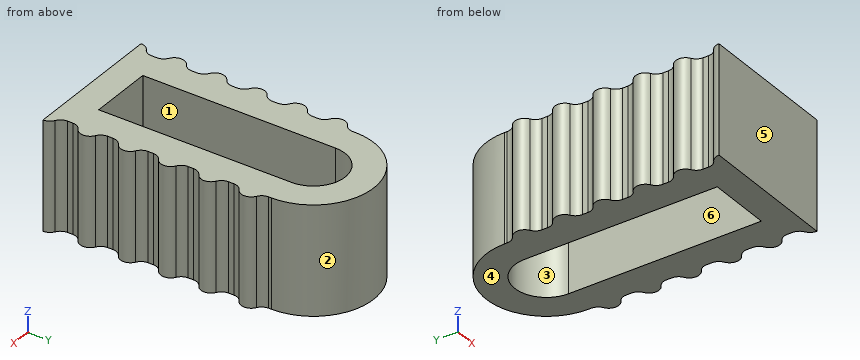
Autodesk Inventor part; units mm, degrees
ref_plane "Plan de construction1" through (3.5, 4, -2.7) normal (0, -1, 0) x (1, 0, 0)
ref_plane "YZ Plane" through (0, 0, 0) normal (1, 0, 0) x (0, 1, 0)
ref_plane "XZ Plane" through (0, 0, 0) normal (0, 1, 0) x (-1, 0, 0)
sketch "Esquisse1" plane through (0, 0, 0) normal (0, 0, 1) x (1, 0, 0)
  line L0 (-3, -7) -> (3, -7)
  line L1 (3, -7) -> (3, 4)
  line L2 (0, 7) -> (0, 7)
  line L3 (-3, 4) -> (-3, -7)
  line L4 (-3, -7) -> (3, 7) construction
  line L5 (3, -7) -> (-3, 7) construction
  arc A0 (0, 7) -> (-3, 4) centre (0, 4) ccw
  arc A1 (3, 4) -> (0, 7) centre (0, 4) ccw
  point P0 (0, 0)
  dimension "d0" = 6
  dimension "d1" = 14
  dimension "d2" = 3
extrude "Extrusion1" add sketch "Esquisse1" along normal mid plane 5.4
sketch "Esquisse2" plane through (0, 0, 2.7) normal (0, 0, 1) x (1, 0, 0)
  line L0 (-3, -7) -> (3, -7) construction
  line L1 (3, -7) -> (3, 4) construction
  arc A0 (3, 4) -> (-3, 4) centre (0, 4) ccw construction
  line L2 (-3, 4) -> (-3, -7) construction
  arc A1 (1.575, 4) -> (-1.575, 4) centre (0, 4) ccw
  line L3 (1.575, 4) -> (1.575, -5.575)
  line L4 (1.575, -5.575) -> (-1.575, -5.575)
  line L5 (-1.575, -5.575) -> (-1.575, 4)
  point P0 (0, 0)
  dimension "d21" = 3.15
extrude "Extrusion2" cut sketch "Esquisse2" against normal through all
sketch "Esquisse3" plane through (0, 0, 2.7) normal (0, 0, 1) x (1, 0, 0)
  line L0 (3, 4) -> (3, -7)
  arc A0 (3.5, -7) -> (3, -6.5) centre (3, -7) ccw
  line L1 (-3, -7) -> (3, -7)
  line L2 (3, -7) -> (3.5, -7)
  line L3 (3, -7) -> (3, -6.5)
  arc A1 (3, -5.5) -> (3, -4.5) centre (3, -5) ccw
  arc A2 (3, -3.5) -> (3, -2.5) centre (3, -3) ccw
  arc A3 (3, -1.5) -> (3, -0.5) centre (3, -1) ccw
  arc A4 (3, 0.5) -> (3, 1.5) centre (3, 1) ccw
  arc A5 (3, 2.5) -> (3, 3.5) centre (3, 3) ccw
  line L4 (3, -5.5) -> (3, -4.5)
  line L5 (3, -3.5) -> (3, -2.5)
  line L6 (3, -1.5) -> (3, -0.5)
  line L7 (3, 0.5) -> (3, 1.5)
  line L8 (3, 2.5) -> (3, 3.5)
  point P0 (0, 0)
  dimension "d8" = 1
  dimension "d9" = 1
  dimension "d10" = 2
  dimension "d13" = 2
extrude "Extrusion3" add sketch "Esquisse3" against normal up to surface (5.4 mm away)
mirror "Symétrie1" about plane through (0, 0, 0) normal (1, 0, 0) of "Extrusion3"
fillet "Congé1" radius 0.5 33 edges at (3, -6.5, -1.35) (3, -6.5, 1.35) (3, -5.5, -1.35) (3, -4.5, -1.35) (3, -5.5, 1.35) (3, -4.5, 1.35) (3, -3.5, -1.35) (3, -2.5, -1.35) (3, -3.5, 1.35) (3, -2.5, 1.35) (3, -1.5, -1.35) (3, -0.5, -1.35) (3, -1.5, 1.35) (3, -0.5, 1.35) (3, 0.5, -1.35) (3, 1.5, -1.35) (3, 0.5, 1.35) (3, 1.5, 1.35) (3, 2.5, -1.35) (3, 3.5, -1.35) (3, 2.5, 1.35) (3, 3.5, 1.35) (-3, -6.5, 0) (-3, -4.5, 0) (-3, -5.5, 0) (-3, -2.5, 0) (-3, -3.5, 0) (-3, -0.5, 0) (-3, -1.5, 0) (-3, 1.5, 0) (-3, 0.5, 0) (-3, 3.5, 0) (-3, 2.5, 0)
ref_plane "Plan de construction1" through (3.5, 4, -2.7) normal (0, -1, 0) x (1, 0, 0)
equation "\"d9\" = d8"
properties part number "Tendeur" material "Aluminium"
Geometry check sheet. Reference: the model listing, model coordinates, mm. Face numbers are marked on the shaded views. A direction names the side the tool comes from. Give positions to 0.01 mm unless a question says otherwise; leave off trailing zeros. Order: outer loops, then holes, each group sorted by start corner. A loop starts at its lowest first (then second) coordinate and runs counter-clockwise, first axis right, second up. Notation, with made-up numbers: (-23.75, -40) - (16.25, -40) arc R15 ccw to (16.25, -13) - close; hole circle Ø7 at (-29.75, 8.5). An arc over 180 degrees is marked (long way). Write item = value, one per line. Start each with the question number.
1) Scan lines: L1, parallel to Y at x = 0, z = 2.35 (3 decimals); L2, parallel to Y at x = 3.25, z = 0.8; L3, parallel to X at y = -5, z = -1.4 (3 decimals). Record each from-to range of solid material in increasing order.
2) Section check D-D (x = 2). Enter the section's corners in (y, z), then the cut area to 3 significant figures.
3) Section check C-C (x = -2.5). Enter the section's corners in (y, z), then the cut area to 3 significant figures.
4) Section check B-B (x = 0). Enter the section's corners in (y, z) (3 decimals), then the cut area to 3 significant figures.
5) Access from +Z, -Z, +X, -X, +Y, -Y to the whole of each face (thin tool, end or side, straight path). Record for the marked faces 1 and 2.
6) Section check A-A (y = 3.25). Enter the section's corners in (x, z) (3 decimals).
7) Draft check along Y on the marked faces 3, 4, 5 and 6. Enter one of: released by +Y, released by -Y, zero draft, split by the parting line, or undercut.
Geometry check:
q1.L1 = -7 to -5.575, 5.575 to 7
q1.L2 = -7 to -6.57, -5.43 to -4.57, -3.43 to -2.57, -1.43 to -0.57, 0.57 to 1.43, 2.57 to 3.43
q1.L3 = -3.5 to -1.575, 1.575 to 3.5
q2.outline = (-7, -2.7) - (6.24, -2.7) - (6.24, 2.7) - (-7, 2.7) - close
q2.area = 71.5 mm2
q3.outline = (-7, -2.7) - (5.66, -2.7) - (5.66, 2.7) - (-7, 2.7) - close
q3.area = 68.4 mm2
q4.outline = (-7, -2.7) - (-5.575, -2.7) - (-5.575, 2.7) - (-7, 2.7) - close; (5.575, -2.7) - (7, -2.7) - (7, 2.7) - (5.575, 2.7) - close
q4.area = 15.4 mm2
q5.face_1 = +Z, -Z
q5.face_2 = +Z, -Z, +Y
q6.outline = (-3.433, -2.7) - (-1.575, -2.7) - (-1.575, 2.7) - (-3.433, 2.7) - close; (1.575, -2.7) - (3.433, -2.7) - (3.433, 2.7) - (1.575, 2.7) - close
q7.face_3 = undercut
q7.face_4 = zero draft
q7.face_5 = released by -Y
q7.face_6 = undercut
